Could you check a few things on this model? Use its own coordinates, in mm. Face numbers are marked on the shaded views. A direction names the side the tool comes from. Give positions to 0.01 mm unless a question says otherwise; leave off trailing zeros. Write each loop counter-clockwise with the first axis right and the second up, starting at its lowest first coordinate (ties: lowest second). Pieces come first, ordered by that corner, then holes. Notation, with made-up numbers: (22, 42) - (50, 42) arc R14 cw to (50, 46) - close; hole circle Ø6 at (50, 26). An arc over 180 degrees is marked (long way). Use one line per item in the form item = value.
```python
from build123d import *
from build123d.topology import SkipClean

# Parameters (mm, degrees)
BOSS_EXTRUDE1_START       = -35
BOSS_EXTRUDE1_OUTLINE_R   = 20
BOSS_EXTRUDE1_OUTLINE_R_2 = 10
BOSS_EXTRUDE1_DEPTH       = 70
BOSS_EXTRUDE2_DEPTH       = 40
SKETCH1_7_W               = 20
SKETCH1_7_H               = 20
BOSS_EXTRUDE3_DEPTH       = 25
BOSS_EXTRUDE4_DEPTH       = 28
SKETCH4_R                 = 28
SKETCH4_R_2               = 10
BOSS_EXTRUDE5_DEPTH       = 60
BOSS_EXTRUDE7_START       = -17.5
BOSS_EXTRUDE7_OUTLINE_R   = 7.5
BOSS_EXTRUDE7_DEPTH       = 35
BOSS_EXTRUDE6_DEPTH       = 28
CUT_EXTRUDE3_DEPTH        = 83
CUT_EXTRUDE3_DEPTH_BACK   = 100
SKETCH8_R                 = 7.5
CUT_EXTRUDE4_DEPTH        = 46
FILLET1_R                 = 10


# Read off the part's stored shape, not the designer's step: Boss-Extrude1, Boss-Extrude7
with BuildPart() as part:
    # Boss-Extrude1 outline → Boss-Extrude1 (new body)
    with BuildSketch(Plane.XY.offset(BOSS_EXTRUDE1_START)):
        with Locations((-110, 0)):
            Circle(BOSS_EXTRUDE1_OUTLINE_R)
        with Locations((-110, 0)):
            Circle(BOSS_EXTRUDE1_OUTLINE_R_2, mode=Mode.SUBTRACT)
    extrude(amount=BOSS_EXTRUDE1_DEPTH)



with BuildPart() as body_2:
    # Sketch1<6> → Boss-Extrude2 (new, symmetric)
    with BuildSketch(Plane.XY):
        with BuildLine():
            ThreePointArc((-50, 0), (0, 50), (50, 0))
            Line((50, 0), (60, 0))
            ThreePointArc((60, 0), (59.135913579, 10.146118724), (56.568542495, 20))
            ThreePointArc((56.568542495, 20), (38.749299446, 45.8092981), (10.342399193, 59.101901652))
            ThreePointArc((10.342399193, 59.101901652), (-38.596995015, 45.937696675), (-60, 0))
            Line((-60, 0), (-50, 0))
        make_face()
    extrude(amount=BOSS_EXTRUDE2_DEPTH, both=True)

    # Sketch1<7> → Boss-Extrude3 (add, symmetric)
    with BuildSketch(Plane.XY):
        with BuildLine():
            ThreePointArc((56.568542495, 20), (59.135913579, 10.146118724), (60, 0))
            Line((60, 0), (80, 0))
            Line((80, 0), (80, 20))
            Line((80, 20), (56.568542495, 20))
        make_face()
        with Locations((90, 10)):
            Rectangle(SKETCH1_7_W, SKETCH1_7_H)
    extrude(amount=BOSS_EXTRUDE3_DEPTH, both=True)


with BuildPart() as part_1:
    add(part.part)

    add(body_2.part)  # Boss-Extrude4 merges body 2
    # Sketch1<10> → Boss-Extrude4 (add, symmetric)
    with BuildSketch(Plane.XY):
        with BuildLine():
            Line((-90, 0), (-70, 0))
            ThreePointArc((-70, 0), (-68.738635424, 13.228756555), (-65, 25.980762114))
            Line((-65, 25.980762114), (-65, 40.311288741))
            ThreePointArc((-65, 40.311288741), (-76.823843083, 19.065374102), (-101.111111111, 17.91612833))
            ThreePointArc((-101.111111111, 17.91612833), (-93.003268288, 10.540925534), (-90, 0))
        make_face()
        with BuildLine():
            Line((-70, 0), (-60, 0))
            ThreePointArc((-60, 0), (-38.596995015, 45.937696675), (10.342399193, 59.101901652))
            ThreePointArc((10.342399193, 59.101901652), (-0.830275834, 62.694222351), (-10.603119378, 69.192296244))
            ThreePointArc((-10.603119378, 69.192296244), (-21.865731835, 66.497291458), (-32.529894875, 61.982303438))
            ThreePointArc((-32.529894875, 61.982303438), (-36.01103024, 60.026708231), (-39.375, 57.87580993))
            ThreePointArc((-39.375, 57.87580993), (-54.569759712, 43.842232208), (-65, 25.980762114))
            ThreePointArc((-65, 25.980762114), (-68.738635424, 13.228756555), (-70, 0))
        make_face()
        with BuildLine():
            Line((-65, 40.311288741), (-65, 25.980762114))
            ThreePointArc((-65, 25.980762114), (-54.569759712, 43.842232208), (-39.375, 57.87580993))
            ThreePointArc((-39.375, 57.87580993), (-49.677071733, 57.304948012), (-55, 66.143782777))
            Line((-55, 66.143782777), (-55, 136))
            Line((-55, 136), (-65, 136))
            Line((-65, 136), (-65, 40.311288741))
        make_face()
        with BuildLine():
            ThreePointArc((-32.529894875, 61.982303438), (-21.865731835, 66.497291458), (-10.603119378, 69.192296244))
            ThreePointArc((-10.603119378, 69.192296244), (-21.234787758, 83.633268621), (-25, 101.166016053))
            Line((-25, 101.166016053), (-25, 136))
            Line((-25, 136), (-35, 136))
            Line((-35, 136), (-35, 101.166016053))
            ThreePointArc((-35, 101.166016053), (-33.329691901, 88.00274883), (-28.424640616, 75.67383951))
            ThreePointArc((-28.424640616, 75.67383951), (-27.598335088, 67.964855653), (-32.529894875, 61.982303438))
        make_face()
    extrude(amount=BOSS_EXTRUDE4_DEPTH, both=True)



with BuildPart() as body_2_2:
    # Sketch4 → Boss-Extrude5 (new body)
    with BuildSketch(Plane(origin=(-15, 0, 0), x_dir=(0, 0, -1), z_dir=(1, 0, 0))):
        with Locations(Location((0, 150, 0), (0, 0, 90))):
            Circle(SKETCH4_R)
        with Locations(Location((0, 150, 0), (0, 0, 90))):
            Circle(SKETCH4_R_2, mode=Mode.SUBTRACT)
    extrude(amount=-BOSS_EXTRUDE5_DEPTH)

    # Boss-Extrude7 outline → Boss-Extrude7 (add)
    with BuildSketch(Plane.XY.offset(BOSS_EXTRUDE7_START)):
        with BuildLine():
            Line((-30, 150), (-30, 190))
            ThreePointArc((-30, 190), (-45, 205), (-60, 190))
            Line((-60, 190), (-60, 150))
            Line((-60, 150), (-30, 150))
        make_face()
        with Locations((-45, 190)):
            Circle(BOSS_EXTRUDE7_OUTLINE_R, mode=Mode.SUBTRACT)
    extrude(amount=BOSS_EXTRUDE7_DEPTH)


with BuildPart() as part_2:
    add(part_1.part)

    add(body_2_2.part)  # Boss-Extrude6 merges body 2 2
    # Sketch1<11> → Boss-Extrude6 (add, symmetric)
    with BuildSketch(Plane.XY):
        Polygon((-35, 136), (-25, 136), (-25, 150), (-30, 150), (-35, 150), align=None)
        Polygon((-65, 150), (-65, 136), (-55, 136), (-55, 150), (-60, 150), align=None)
    extrude(amount=BOSS_EXTRUDE6_DEPTH, both=True)

    # Sketch7 → Cut-Extrude3 (cut, two sides: drawn at the far end of the back side and taken through both)
    with SkipClean():  # the faces are left unmerged after this step: merging them gives an invalid solid
        with BuildSketch(Plane(origin=(-25, 0, 0), x_dir=(0, 0, -1), z_dir=(1, 0, 0)).offset(-CUT_EXTRUDE3_DEPTH_BACK)):
            with BuildLine():
                ThreePointArc((2.5, 159.682458366), (1.260042925, 159.920296963), (0, 160))
                ThreePointArc((0, 160), (-1.260042925, 159.920296963), (-2.5, 159.682458366))
                ThreePointArc((-2.5, 159.682458366), (-7.90569415, 156.123724357), (-10, 150))
                Line((-10, 150), (10, 150))
                ThreePointArc((10, 150), (7.90569415, 156.123724357), (2.5, 159.682458366))
            make_face()
            with BuildLine():
                ThreePointArc((-10, 150), (0, 140), (10, 150))
                Line((10, 150), (-10, 150))
            make_face()
            with BuildLine():
                Line((0, 205), (0, 160))
                ThreePointArc((0, 160), (1.260042925, 159.920296963), (2.5, 159.682458366))
                Line((2.5, 159.682458366), (2.5, 205))
                Line((2.5, 205), (0, 205))
            make_face()
            with BuildLine():
                ThreePointArc((-2.5, 159.682458366), (-1.260042925, 159.920296963), (0, 160))
                Line((0, 160), (0, 205))
                Line((0, 205), (-2.5, 205))
                Line((-2.5, 205), (-2.5, 159.682458366))
            make_face()
        extrude(amount=CUT_EXTRUDE3_DEPTH + CUT_EXTRUDE3_DEPTH_BACK, mode=Mode.SUBTRACT)

    # Sketch8 → Cut-Extrude4 (cut)
    with SkipClean():  # the faces are left unmerged after this step: merging them gives an invalid solid
        with BuildSketch(Plane(origin=(0, 20, 0), x_dir=(1, 0, 0), z_dir=(0, 1, 0))):
            with Locations(Location((80, 0, 0), (0, 0, 180))):
                Circle(SKETCH8_R)
        extrude(amount=-CUT_EXTRUDE4_DEPTH, mode=Mode.SUBTRACT)

    # Fillet1
    fillet1_edges = [part_2.edges().sort_by_distance(p)[0] for p in [
        (100, 10, -25),
        (100, 10, 25),
    ]]
    fillet(fillet1_edges, radius=FILLET1_R)


solid = part_2.part
```
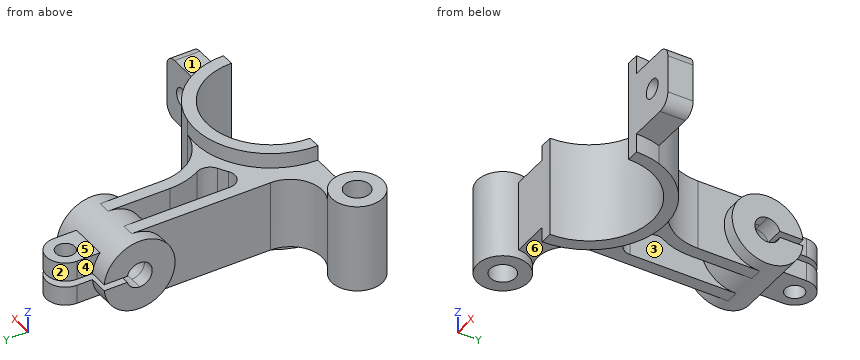
1. If we mould it in two halves opening along X, with no side actions, what happens to the marked faces 1, 2 and 3? For each: pulls with the +X half, pulls with the -X half, needs draft (parallel to the pull), parting line crosses it, or undercut.
Response values:
face_1 = needs draft
face_2 = parting line crosses it
face_3 = undercut
2. Imagine slicing it at D-D, the plane x = 0. List the corners of the cut face in (y, z) for me.
Response values:
outline = (50, -40) - (60, -40) - (60, -28) - (62.31, -28) - (62.31, 28) - (60, 28) - (60, 40) - (50, 40) - close
3. For pin 1 (3 mm diameter, centred on x = -86, z = 25.5, fed in from +Y); pin 2 (6 mm diameter, centred on x = 56, z = -13, fed in from -Y); pin 3 (16 mm diameter, centred on x = -110, y = 0, fed in from +Z); pin 4 (20 mm diameter, centred on x = -113.5, y = -4, fed in from -Z), each with a flat end and sliding along its axis, tell me the tip position at first contact or that it passes through.
Response values:
pin_1 = 15.92
pin_2 = 0
pin_3 = through
pin_4 = -35
4. Imagine slicing it at A-A, the plane x = -110. List the corners of the cut face in (y, z) for me.
Response values:
outline = (-20, -35) - (-10, -35) - (-10, 35) - (-20, 35) - close; (10, -35) - (20, -35) - (20, 35) - (10, 35) - close
5. Imagine slicing it at C-C, the plane x = -45. List the corners of the cut face in (y, z) for me.
Response values:
outline = (21.79, -40) - (39.69, -40) - (39.69, -28) - (56.14, -28) - (56.14, 28) - (39.69, 28) - (39.69, 40) - (21.79, 40) - close; (159.68, -2.5) arc R10 cw (long way) to (159.68, 2.5) - (182.5, 2.5) - (182.5, 17.5) - (171.86, 17.5) arc R28 ccw (long way) to (171.86, -17.5) - (182.5, -17.5) - (182.5, -2.5) - close; (197.5, -17.5) - (205, -17.5) - (205, -2.5) - (197.5, -2.5) - close; (197.5, 2.5) - (205, 2.5) - (205, 17.5) - (197.5, 17.5) - close
6. If I drill on line 1 (Y direction, x = -45, z = 13); line 2 (Z direction, x = 80, y = 13.75); line 3 (Y direction, x = -110, z = 4.5), over which ranges is the centre line in solid material (lowest first)? Write a range as from..to.
Response values:
line_1 = 21.79..56.14, 125.2..182.5, 197.5..205
line_2 = -25..-7.5, 7.5..25
line_3 = -20..-10, 10..20
7. Which directions (+Z, -Z, +X, -X, +Y, -Y) give clear straight access to the entire face, cutting with the end or side of a thin tool? Please do the marked faces 4, 5 and 6.
Response values:
face_4 = +Z, -X, +Y
face_5 = +Z, +X, -X, +Y
face_6 = -Z, +Y
8. Imagine slicing it at B-B, the plane y = 108. List the corners of the cut face in (x, z) for me, and give its area (3 significant figures).
Response values:
outline = (-65, -28) - (-55, -28) - (-55, 28) - (-65, 28) - close; (-35, -28) - (-25, -28) - (-25, 28) - (-35, 28) - close
area = 1,120 mm²
